Work out the finished part from the listing and answer in its coordinate system (mm). Face numbers are marked on the shaded views. A direction names the side the tool comes from. Give positions to 0.01 mm unless a question says otherwise; leave off trailing zeros. Order: outer loops, then holes, each group sorted by start corner. A loop starts at its lowest first (then second) coordinate and runs counter-clockwise, first axis right, second up. Notation, with made-up numbers: (76.5, 66) -> (128.5, 66) arc R18 cw to (128.5, 89) -> close; hole circle Ø9 at (55, 30.25). An arc over 180 degrees is marked (long way). Use a Markdown table: item, result. Add a question column.
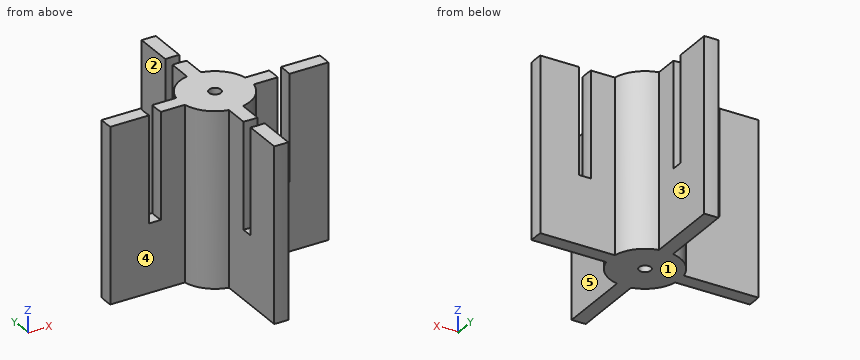
```python
from build123d import *

# Parameters (mm, degrees)
SKETCH1_R           = 46.5
BOSS_EXTRUDE1_DEPTH = 74
SKETCH2_R           = 2.5
CUT_EXTRUDE1_DEPTH  = 10
SKETCH3_R           = 2.5
CUT_EXTRUDE2_DEPTH  = 10
SKETCH4_OUTSIDE_W   = 125.182
SKETCH4_OUTSIDE_H   = 125.182
CUT_EXTRUDE3_DEPTH  = 75
SKETCH7_R           = 30
SKETCH7_R_2         = 25
CUT_EXTRUDE4_DEPTH  = 45


with BuildPart() as part:
    # Sketch1 → Boss-Extrude1 (new body)
    with BuildSketch(Plane.XY):
        Circle(SKETCH1_R)
    extrude(amount=BOSS_EXTRUDE1_DEPTH)

    # Sketch2 → Cut-Extrude1 (cut)
    with BuildSketch(Plane.XY.offset(74)):
        Circle(SKETCH2_R)
    extrude(amount=-CUT_EXTRUDE1_DEPTH, mode=Mode.SUBTRACT)

    # Sketch3 → Cut-Extrude2 (cut)
    with BuildSketch(Plane(origin=(0, 0, 0), x_dir=(-1, 0, 0), z_dir=(0, 0, -1))):
        Circle(SKETCH3_R)
    extrude(amount=-CUT_EXTRUDE2_DEPTH, mode=Mode.SUBTRACT)

    # Sketch4 outside → Cut-Extrude3 (cut, through all)
    with BuildSketch(Plane(origin=(0, 0, 0), x_dir=(-1, 0, 0), z_dir=(0, 0, -1))):
        Rectangle(SKETCH4_OUTSIDE_W, SKETCH4_OUTSIDE_H)
        with BuildLine():
            Line((-46.403124895, 3), (-14.696938457, 3))
            ThreePointArc((-14.696938457, 3), (-10.606601718, 10.606601718), (-3, 14.696938457))
            Line((-3, 14.696938457), (-3, 46.403124895))
            ThreePointArc((-3, 46.403124895), (0, 46.5), (3, 46.403124895))
            Line((3, 46.403124895), (3, 14.696938457))
            ThreePointArc((3, 14.696938457), (10.606601718, 10.606601718), (14.696938457, 3))
            Line((14.696938457, 3), (46.403124895, 3))
            ThreePointArc((46.403124895, 3), (46.5, 0), (46.403124895, -3))
            Line((46.403124895, -3), (14.696938457, -3))
            ThreePointArc((14.696938457, -3), (10.606601718, -10.606601718), (3, -14.696938457))
            Line((3, -14.696938457), (3, -46.403124895))
            ThreePointArc((3, -46.403124895), (0, -46.5), (-3, -46.403124895))
            Line((-3, -46.403124895), (-3, -14.696938457))
            ThreePointArc((-3, -14.696938457), (-10.606601718, -10.606601718), (-14.696938457, -3))
            Line((-14.696938457, -3), (-46.403124895, -3))
            ThreePointArc((-46.403124895, -3), (-46.5, 0), (-46.403124895, 3))
        make_face(mode=Mode.SUBTRACT)
    extrude(amount=-CUT_EXTRUDE3_DEPTH, mode=Mode.SUBTRACT)

    # Sketch7 → Cut-Extrude4 (cut)
    with BuildSketch(Plane.XY.offset(74)):
        Circle(SKETCH7_R)
        Circle(SKETCH7_R_2, mode=Mode.SUBTRACT)
    extrude(amount=-CUT_EXTRUDE4_DEPTH, mode=Mode.SUBTRACT)


solid = part.part
```
1) Flat-ended cylindrical pins translate along their axes: pin 1 (8 mm diameter, centred on y = -9, z = 46.5, fed in from +X); pin 2 (4 mm diameter, centred on x = 1.5, y = 27, fed in from +Z); pin 3 (12 mm diameter, centred on x = 25, z = 16.5, fed in from +Y). Find the tip coordinate at first contact, or state that the pin passes through.
2) The part is cut by section A-A, the plane z = 48. State how many separate pieces and enclosed holes the cut face has, then the cut area to 3 significant figures.
3) The part is cut by section B-B, the plane x = 0. Determine the outline of the cut face in (y, z), then the cut area to 3 significant figures.
4) Straight lines are drawn through the part: line 1 (Y direction, x = 0, z = 69); line 2 (Y direction, x = 0, z = 5); line 3 (Y direction, x = -1.5, z = 33). For each, find the intervals that lie inside material, in ascending order.
5) Which of the six approach directions +Z, -Z, +X, -X, +Y, -Y give full straight-line access (tool end or side, diameter ignored) to the marked faces 1, 2, 3, 4 and 5?
6) The part is cut by section D-D, the plane z = 20. Determine the outline of the cut face in (x, y).
A:
| question | item | result |
|---|---|---|
| 1 | pin 1 | x = 14.14 |
| 1 | pin 2 | z = 29 |
| 1 | pin 3 | y = 3 |
| 2 | separate pieces | 5 |
| 2 | enclosed holes | 0 |
| 2 | area | 1,340 mm^2 |
| 3 | outline | (-46.5, 0) -> (-2.5, 0) -> (-2.5, 10) -> (2.5, 10) -> (2.5, 0) -> (46.5, 0) -> (46.5, 74) -> (30, 74) -> (30, 29) -> (25, 29) -> (25, 74) -> (2.5, 74) -> (2.5, 64) -> (-2.5, 64) -> (-2.5, 74) -> (-25, 74) -> (-25, 29) -> (-30, 29) -> (-30, 74) -> (-46.5, 74) -> close |
| 3 | area | 6,330 mm^2 |
| 4 | line 1 | -46.5 to -30, -25 to -2.5, 2.5 to 25, 30 to 46.5 |
| 4 | line 2 | -46.5 to -2.5, 2.5 to 46.5 |
| 4 | line 3 | -46.48 to -29.96, -24.95 to 24.95, 29.96 to 46.48 |
| 5 | face 1 | -Z, +X, -X, +Y, -Y |
| 5 | face 2 | +Z, -Z, -X, +Y |
| 5 | face 3 | +Z, -Z, +X, +Y |
| 5 | face 4 | +Z, -Z, -X, -Y |
| 5 | face 5 | +Z, -Z, +X, -Y |
| 6 | outline | (-46.4, -3) -> (-14.7, -3) arc R15 ccw to (-3, -14.7) -> (-3, -46.4) arc R46.5 ccw to (3, -46.4) -> (3, -14.7) arc R15 ccw to (14.7, -3) -> (46.4, -3) arc R46.5 ccw to (46.4, 3) -> (14.7, 3) arc R15 ccw to (3, 14.7) -> (3, 46.4) arc R46.5 ccw to (-3, 46.4) -> (-3, 14.7) arc R15 ccw to (-14.7, 3) -> (-46.4, 3) arc R46.5 ccw to start |
